Answer from the drawing. Dimensions are ordinates in mm from the lowest x, y and z of the part. Round coordinates to 2 decimals unless told otherwise and drop trailing zeros. Loops run counter-clockwise (first coordinate to the right, second up) from the corner with the lowest first, then second, coordinate; pieces in that order, holes last.
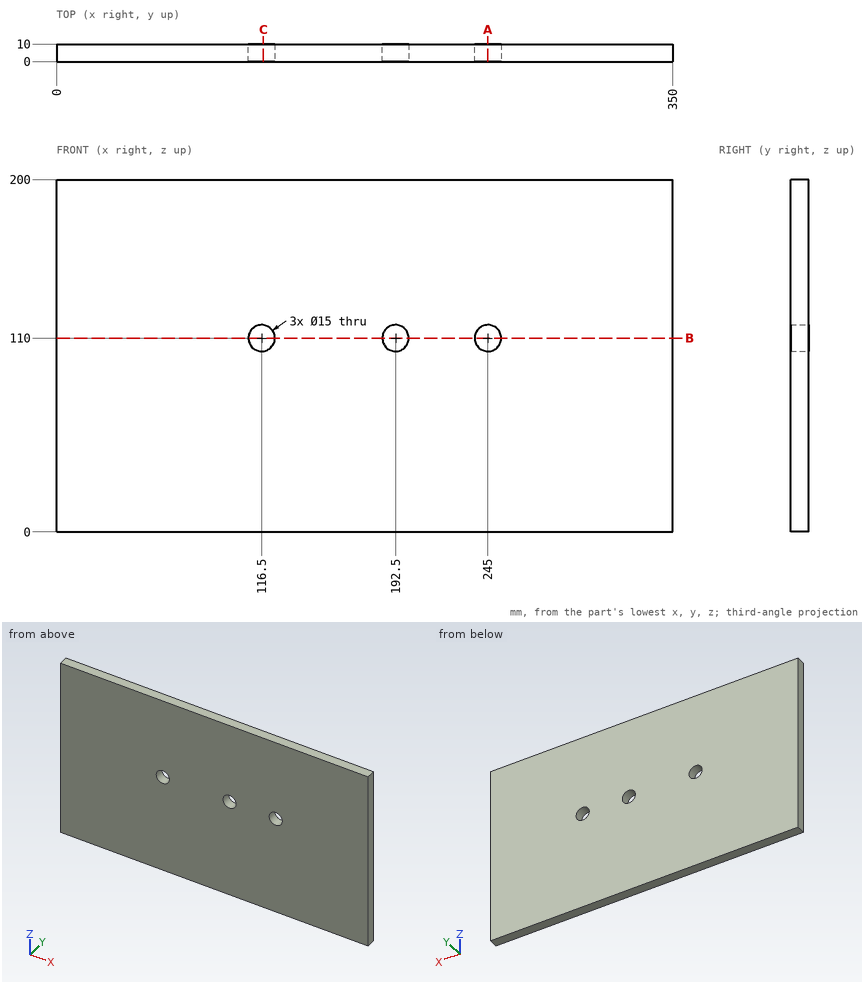
1. Find section B-B (z = 110). Write down the section's boundary in (x, y), then the cut area to 3 significant figures.
Answer key:
outline: (0, 0) - (109, 0) - (109, 10) - (0, 10) - close; (124, 0) - (185, 0) - (185, 10) - (124, 10) - close; (200, 0) - (237.5, 0) - (237.5, 10) - (200, 10) - close; (252.5, 0) - (350, 0) - (350, 10) - (252.5, 10) - close
area: 3,050 mm2
2. Find section C-C (x = 117.5). Write down the section's boundary in (y, z).
Answer key:
outline: (0, 0) - (10, 0) - (10, 102.57) - (0, 102.57) - close; (0, 117.43) - (10, 117.43) - (10, 200) - (0, 200) - close
3. Find section A-A (x = 245). Write down the section's boundary in (y, z), then the cut area to 3 significant figures.
Answer key:
outline: (0, 0) - (10, 0) - (10, 102.5) - (0, 102.5) - close; (0, 117.5) - (10, 117.5) - (10, 200) - (0, 200) - close
area: 1,850 mm2
4. Consider probe 1 along Z at (x, y) = (116.5, 6); probe 2 along X at (y, z) = (2.5, 116.5); probe 3 along Z at (x, y) = (198.5, 5). Determine where each line is inside the solid, lowest interval first.
Answer key:
probe 1: z = 0 to 102.5, 117.5 to 200
probe 2: x = 0 to 112.76, 120.24 to 188.76, 196.24 to 241.26, 248.74 to 350
probe 3: z = 0 to 105.5, 114.5 to 200
